Geometry: final body of the model. Coordinates: model frame, mm. Face numbers are marked on the shaded views. A direction names the side the tool comes from. Round coordinates to 2 decimals unless told otherwise and drop trailing zeros. Loops run counter-clockwise (first coordinate to the right, second up) from the corner with the lowest first, then second, coordinate; pieces in that order, holes last. Notation, with made-up numbers: M 79,-16 L 133,-16 A17 ccw 133,15 Z; hole C 14,35 d6. An arc over 180 degrees is marked long. Answer as a JSON object with one key per item and string values.
from build123d import *

# Parameters (mm, degrees)
SKETCH1_R           = 1.75
BOSS_EXTRUDE1_DEPTH = 5
SKETCH2_W           = 100
SKETCH2_H           = 38
BOSS_EXTRUDE2_DEPTH = 14
SKETCH3_W           = 50
SKETCH3_H           = 5
BOSS_EXTRUDE3_DEPTH = 15
SKETCH4_R           = 1.75
CUT_EXTRUDE1_DEPTH  = 16
BOSS_EXTRUDE6_DEPTH = 15
SKETCH9_R           = 3.25
CUT_EXTRUDE3_DEPTH  = 36
SKETCH10_R          = 5.25
CUT_EXTRUDE4_DEPTH  = 9
CUT_EXTRUDE5_REACH  = 28.5
SKETCH11_W          = 5
SKETCH11_H          = 9.2
SKETCH12_R          = 1.75
CUT_EXTRUDE6_DEPTH  = 4
SKETCH13_W          = 100
SKETCH13_H          = 13
BOSS_EXTRUDE7_DEPTH = 30
SKETCH14_R          = 2.5
CUT_EXTRUDE7_DEPTH  = 39
CUT_EXTRUDE8_DEPTH  = 4
SKETCH16_R          = 2.1
CUT_EXTRUDE9_DEPTH  = 4
CHAMFER1_SIZE       = 1.6
CUT_EXTRUDE10_DEPTH = 39
CHAMFER2_SIZE       = 1.6
CHAMFER3_SIZE       = 5
SKETCH18_R          = 1.75
CUT_EXTRUDE11_DEPTH = 4
FILLET1_R           = 5
FILLET2_R           = 2
FILLET3_R           = 4


with BuildPart() as part:
    # Sketch1 → Boss-Extrude1 (new body)
    with BuildSketch(Plane(origin=(0, 0, 0), x_dir=(1, 0, 0), z_dir=(0, 1, 0))):
        Polygon((-10, 50), (10, 50), (11, 50), (11, -50), (10, -50), (-10, -50), align=None)
        with Locations((-7.5, 36)):
            Circle(SKETCH1_R, mode=Mode.SUBTRACT)
        with Locations((7.5, 36)):
            Circle(SKETCH1_R, mode=Mode.SUBTRACT)
        with Locations((-7.5, 20)):
            Circle(SKETCH1_R, mode=Mode.SUBTRACT)
        with Locations((7.5, 20)):
            Circle(SKETCH1_R, mode=Mode.SUBTRACT)
        with Locations((7.5, -20)):
            Circle(SKETCH1_R, mode=Mode.SUBTRACT)
        with Locations((-7.5, -20)):
            Circle(SKETCH1_R, mode=Mode.SUBTRACT)
        with Locations((7.5, -36)):
            Circle(SKETCH1_R, mode=Mode.SUBTRACT)
        with Locations((-7.5, -36)):
            Circle(SKETCH1_R, mode=Mode.SUBTRACT)
    extrude(amount=BOSS_EXTRUDE1_DEPTH)

    # Sketch2 → Boss-Extrude2 (add)
    with BuildSketch(Plane(origin=(11, 0, 0), x_dir=(0, 0, -1), z_dir=(1, 0, 0))):
        with Locations((0, -14)):
            Rectangle(SKETCH2_W, SKETCH2_H)
    extrude(amount=BOSS_EXTRUDE2_DEPTH)

    # Sketch3 → Boss-Extrude3 (add)
    with BuildSketch(Plane(origin=(25, 0, 0), x_dir=(0, 0, -1), z_dir=(1, 0, 0))):
        with Locations((0, -20.5)):
            Rectangle(SKETCH3_W, SKETCH3_H)
    extrude(amount=BOSS_EXTRUDE3_DEPTH)

    # Sketch4 → Cut-Extrude1 (cut, through all)
    with BuildSketch(Plane(origin=(0, -18, 0), x_dir=(1, 0, 0), z_dir=(0, 1, 0))):
        with Locations((35, 15)):
            Circle(SKETCH4_R)
        with Locations((35, -15)):
            Circle(SKETCH4_R)
    extrude(amount=-CUT_EXTRUDE1_DEPTH, mode=Mode.SUBTRACT)

    # Sketch8 → Boss-Extrude6 (add)
    with BuildSketch(Plane(origin=(25, 0, 0), x_dir=(0, 0, -1), z_dir=(1, 0, 0))):
        Polygon((-50, -6.5), (-25, -6.5), (-25, -33), (-50, -33), (-50, -30), (-29.5, -30), (-29.5, -9.5), (-50, -9.5), align=None)
        Polygon((29.5, -30), (29.5, -9.5), (50, -9.5), (50, -6.5), (25, -6.5), (25, -33), (50, -33), (50, -30), align=None)
    extrude(amount=BOSS_EXTRUDE6_DEPTH)

    # Sketch9 → Cut-Extrude3 (cut, through all)
    with BuildSketch(Plane(origin=(25, 0, 0), x_dir=(0, 0, -1), z_dir=(1, 0, 0))):
        with Locations((-39.75, -19.75)):
            Circle(SKETCH9_R)
        with Locations((39.75, -19.75)):
            Circle(SKETCH9_R)
    extrude(amount=-CUT_EXTRUDE3_DEPTH, mode=Mode.SUBTRACT)

    # Sketch10 → Cut-Extrude4 (cut)
    with BuildSketch(Plane.ZY.offset(-11)):
        with Locations((-39.75, -19.75)):
            Circle(SKETCH10_R)
        with Locations((39.75, -19.75)):
            Circle(SKETCH10_R)
    extrude(amount=-CUT_EXTRUDE4_DEPTH, mode=Mode.SUBTRACT)

    # Sketch11 → Cut-Extrude5 (cut, up to next)
    with BuildSketch(Plane(origin=(0, -6.5, 0), x_dir=(1, 0, 0), z_dir=(0, 1, 0)), mode=Mode.PRIVATE) as cut_extrude5_sk1:
        with Locations((37.5, -39.75)):
            Rectangle(SKETCH11_W, SKETCH11_H)
    cut_extrude5_tool1 = extrude(cut_extrude5_sk1.sketch, amount=-CUT_EXTRUDE5_REACH, mode=Mode.PRIVATE) & part.part
    add(cut_extrude5_tool1.solids().sort_by_distance((37.5, -6.5, 39.75))[0], mode=Mode.SUBTRACT)
    # Sketch11 → Cut-Extrude5 (cut, up to next)
    with BuildSketch(Plane(origin=(0, -6.5, 0), x_dir=(1, 0, 0), z_dir=(0, 1, 0)), mode=Mode.PRIVATE) as cut_extrude5_sk2:
        with Locations((37.5, 39.75)):
            Rectangle(SKETCH11_W, SKETCH11_H)
    cut_extrude5_tool2 = extrude(cut_extrude5_sk2.sketch, amount=-CUT_EXTRUDE5_REACH, mode=Mode.PRIVATE) & part.part
    add(cut_extrude5_tool2.solids().sort_by_distance((37.5, -6.5, -39.75))[0], mode=Mode.SUBTRACT)

    # Sketch12 → Cut-Extrude6 (cut, through all)
    with BuildSketch(Plane(origin=(0, -30, 0), x_dir=(1, 0, 0), z_dir=(0, 1, 0))):
        with Locations((32.5, -39.75)):
            Circle(SKETCH12_R)
        with Locations((32.5, 39.75)):
            Circle(SKETCH12_R)
    extrude(amount=-CUT_EXTRUDE6_DEPTH, mode=Mode.SUBTRACT)

    # Sketch13 → Boss-Extrude7 (add)
    with BuildSketch(Plane.ZY.offset(10)):
        with Locations((0, -1.5)):
            Rectangle(SKETCH13_W, SKETCH13_H)
    extrude(amount=BOSS_EXTRUDE7_DEPTH)

    # Sketch14 → Cut-Extrude7 (cut, through all)
    with BuildSketch(Plane(origin=(0, 5, 0), x_dir=(1, 0, 0), z_dir=(0, 1, 0))):
        with Locations((-21.15, 28.4925)):
            Circle(SKETCH14_R)
        with Locations((-31.1525, -28.725)):
            Circle(SKETCH14_R)
    extrude(amount=-CUT_EXTRUDE7_DEPTH, mode=Mode.SUBTRACT)

    # Sketch15 → Cut-Extrude8 (cut)
    with BuildSketch(Plane.XZ.offset(8)):
        Polygon((-27.1525, 26.415598923), (-27.1525, 31.034401077), (-31.1525, 33.343802154), (-35.1525, 31.034401077), (-35.1525, 26.415598923), (-31.1525, 24.106197846), align=None)
        Polygon((-25.15, -30.801901077), (-21.15, -33.111302154), (-17.15, -30.801901077), (-17.15, -26.183098923), (-21.15, -23.873697846), (-25.15, -26.183098923), align=None)
    extrude(amount=-CUT_EXTRUDE8_DEPTH, mode=Mode.SUBTRACT)

    # Sketch16 → Cut-Extrude9 (cut)
    with BuildSketch(Plane(origin=(0, 5, 0), x_dir=(1, 0, 0), z_dir=(0, 1, 0))):
        with Locations((20, 39.75)):
            Circle(SKETCH16_R)
        with Locations((20, -39.75)):
            Circle(SKETCH16_R)
    extrude(amount=-CUT_EXTRUDE9_DEPTH, mode=Mode.SUBTRACT)

    # Chamfer1
    chamfer1_edges = [part.edges().sort_by_distance(p)[0] for p in [
        (-9.25, 5, -36),
        (5.75, 5, -36),
        (-9.25, 5, -20),
        (5.75, 5, -20),
        (5.75, 5, 20),
        (-9.25, 5, 20),
        (5.75, 5, 36),
        (-9.25, 5, 36),
    ]]
    chamfer(chamfer1_edges, length=CHAMFER1_SIZE)

    # Sketch17 → Cut-Extrude10 (cut, through all)
    with BuildSketch(Plane(origin=(0, 5, 0), x_dir=(1, 0, 0), z_dir=(0, 1, 0))):
        Polygon((-40, 20), (-15, 7.5), (-15, -7.5), (-40, -20), align=None)
    extrude(amount=-CUT_EXTRUDE10_DEPTH, mode=Mode.SUBTRACT)

    # Chamfer2
    chamfer2_edges = [part.edges().sort_by_distance(p)[0] for p in [
        (30.75, -33, 39.75),
        (30.75, -33, -39.75),
    ]]
    chamfer(chamfer2_edges, length=CHAMFER2_SIZE)

    # Chamfer3
    chamfer3_edges = [part.edges().sort_by_distance(p)[0] for p in [
        (11, -33, 0),
    ]]
    chamfer(chamfer3_edges, length=CHAMFER3_SIZE)

    # Sketch18 → Cut-Extrude11 (cut)
    with BuildSketch(Plane(origin=(0, 1, 0), x_dir=(1, 0, 0), z_dir=(0, 1, 0))):
        with Locations((20, 39.75)):
            Circle(SKETCH18_R)
        with Locations((20, -39.75)):
            Circle(SKETCH18_R)
    extrude(amount=-CUT_EXTRUDE11_DEPTH, mode=Mode.SUBTRACT)

    # Fillet1
    fillet1_edges = [part.edges().sort_by_distance(p)[0] for p in [
        (-40, -1.5, -50),
        (-40, -1.5, 50),
        (-40, -1.5, 20),
        (-40, -1.5, -20),
        (-15, -1.5, -7.5),
        (-15, -1.5, 7.5),
    ]]
    fillet(fillet1_edges, radius=FILLET1_R)

    # Fillet2
    fillet2_edges = [part.edges().sort_by_distance(p)[0] for p in [
        (25, 5, 0),
    ]]
    fillet(fillet2_edges, radius=FILLET2_R)

    # Fillet3
    fillet3_edges = [part.edges().sort_by_distance(p)[0] for p in [
        (32.5, -6.5, -25),
        (32.5, -33, -25),
        (32.5, -33, 25),
        (32.5, -6.5, 25),
    ]]
    fillet(fillet3_edges, radius=FILLET3_R)


solid = part.part
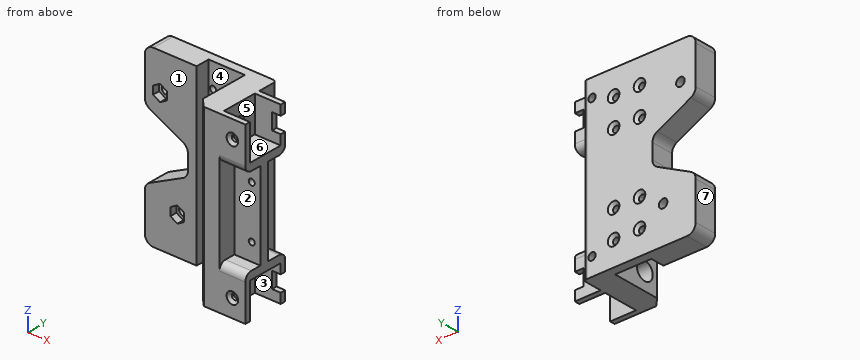
1) Reachability of the marked faces 1, 2 and 3 from +Z, -Z, +X, -X, +Y, -Y: full face, straight path, thin tool, end or side. Return the list, or none.
Results:
{"face 1": "+Z, -Z, -X, -Y", "face 2": "+X, -Y", "face 3": "-Z, +X"}
2) Pin query (flat end, axial travel): P1, Ø3, axis at y = -15.5, z = 2, coming from the -X side; P2, Ø5, axis at y = 0, z = -2, coming from the -X side; P3, Ø10.5, axis at x = -2, z = -15.5, coming from the -Y side. Return the tip coordinate at first contact, or that it passes through.
Results:
{"P1": "x = 11", "P2": "x = -15", "P3": "y = 0"}
3) Ray query, line 1 (Z direction, x = 20, y = -0.45); line 2 (Z direction, x = 21, y = -22); line 3 (X direction, y = 1.95, z = 20). Return the intervals inside material, ascending.
Results:
{"line 1": "-50 to -41.5, -38 to 38, 41.5 to 50", "line 2": "-50 to -42.1, -37.4 to 37.4, 42.1 to 50", "line 3": "-38.93 to -9.25, -5.75 to 5.75, 9.25 to 25"}
4) Pull-direction query (X, two-part tool) for the marked faces 4, 5, 6 and 7; classes: +X half, -X half, draft (parallel to the pull), parting line (faces both ways), or undercut.
Results:
{"face 4": "undercut", "face 5": "+X half", "face 6": "draft", "face 7": "-X half"}
5) Section query C-C (z = 15). Return the cut outline in (x, y).
Results:
{"outline": "M -30,-8 L -10,-8 L -10,0 L 11,0 L 11,-28 L 16,-33 L 25,-33 L 25,-23 L 33.25,-23 L 33.25,-18 L 25,-18 L 25,3 A2 ccw 23,5 L -30,5 Z; M 36.75,-23 L 40,-23 L 40,-18 L 36.75,-18 Z"}
6) Section query B-B (x = 7.5). Return the cut outline in (y, z).
Results:
{"outline": "M 0,-50 L 5,-50 L 5,-39.35 L 3.4,-37.75 L 0,-37.75 Z; M 0,-34.25 L 3.4,-34.25 L 5,-32.65 L 5,-23.35 L 3.4,-21.75 L 0,-21.75 Z; M 0,-18.25 L 3.4,-18.25 L 5,-16.65 L 5,16.65 L 3.4,18.25 L 0,18.25 Z; M 0,21.75 L 3.4,21.75 L 5,23.35 L 5,32.65 L 3.4,34.25 L 0,34.25 Z; M 0,37.75 L 3.4,37.75 L 5,39.35 L 5,50 L 0,50 Z"}
7) Section query A-A (y = -19.75). Return the cut outline in (x, z), and give its area (3 significant figures).
Results:
{"outline": "M 11,-50 L 25,-50 L 25,-43 L 20,-43 L 20,-45 L 11,-45 Z; M 11,-34.5 L 20,-34.5 L 20,-36.5 L 25,-36.5 L 25,-29.5 L 40,-29.5 L 40,29.5 L 25,29.5 L 25,36.5 L 20,36.5 L 20,34.5 L 11,34.5 Z; M 11,45 L 20,45 L 20,43 L 25,43 L 25,50 L 11,50 Z; hole C 35,-15 d3.5; hole C 35,15 d3.5", "area": "2,010 mm2"}
